```python
from build123d import *

# Parameters (mm, degrees)
F0_R     = 15
F1_DEPTH = 20
F2_W     = 40
F2_H     = 40
F3_DEPTH = 100
F5_D     = 17


with BuildPart() as f1:
    # F0 (on Right) → F1 (new body, symmetric)
    with BuildSketch(Plane.YZ):
        Polygon((-80, -5), (-40, -40), (40, -40), (80, -5), (80, 35), (-80, 35), align=None)
        Circle(F0_R, mode=Mode.SUBTRACT)
    extrude(amount=F1_DEPTH, both=True)

    # F2 (on Right) → F3 (join, symmetric)
    with BuildSketch(Plane.YZ):
        with Locations((-60, 15)):
            Rectangle(F2_W, F2_H)
        with Locations((60, 15)):
            Rectangle(F2_W, F2_H)
    extrude(amount=F3_DEPTH, both=True)

    # F5 (through all)
    with Locations(Plane.XY.offset(35)):
        with Locations((-80, 60), (80, 60), (80, -60), (-80, -60)):
            Hole(F5_D / 2)


solid = f1.part
```
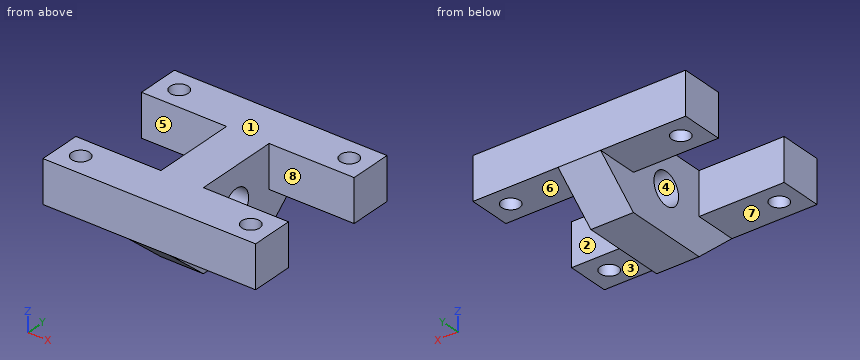
Geometry: final body of the model. Coordinates: model frame, mm. Face numbers are marked on the shaded views. A direction names the side the tool comes from. Round coordinates to 2 decimals unless told otherwise and drop trailing zeros. Order: outer loops, then holes, each group sorted by start corner. A loop starts at its lowest first (then second) coordinate and runs counter-clockwise, first axis right, second up. Notation, with made-up numbers: (34, -5.5) - (44, -5.5) arc R30 cw to (44, 26.5) - close; hole circle Ø1 at (73.25, 82). An arc over 180 degrees is marked (long way). Write item = value, one per line. Start each with the question number.
Q1. Ray query, line 1 (Y direction, x = 80, z = 11); line 2 (Z direction, x = -0.5, y = 0); line 3 (Y direction, x = 70.5, z = 11). Return the intervals inside material, ascending. Write a range as from..to.
Q2. Access query for the marked faces 5, 6, 7 and 8. Directions: +Z, -Z, +X, -X, +Y, -Y. A direction counts if a zero-diameter tool reaches every point of the face in a straight line with its end or side. Return the directions, or none.
Q3. Cut plane D-D on y = 60. Return the cut outline in (x, z), and give its area (3 significant figures).
Q4. Pin query (flat end, axial travel): pin 1 (1.5 mm diameter, centred on y = -38, z = -32, fed in from -X); pin 2 (20 mm diameter, centred on x = -66, y = -65, fed in from -Z); pin 3 (22.5 mm diameter, centred on y = 7, z = 9.5, fed in from +X). Return the tip coordinate at first contact, or that it passes through.
Q5. Pull-direction query (Z, two-part tool) for the marked faces 1, 2, 3 and 4; classes: +Z half, -Z half, draft (parallel to the pull), parting line (faces both ways), or undercut.
Q6. Cut plane A-A on z = 0. Return the cut outline in (x, y).
Q7. Cut plane B-B on y = 0. Return the cut outline in (x, z), and give its area (3 significant figures).
Q8. Cut plane C-C on x = -37. Return the cut outline in (y, z).
Outcome:
q1.line_1 = -80..-68.5, -51.5..-40, 40..51.5, 68.5..80
q1.line_2 = -40..-15, 15..35
q1.line_3 = -80..-40, 40..80
q2.face_5 = +Z, -Z, -X
q2.face_6 = -Z, +X, +Y, -Y
q2.face_7 = -Z, -X, +Y, -Y
q2.face_8 = +Z, -Z, +X
q3.outline = (-100, -5) - (-88.5, -5) - (-88.5, 35) - (-100, 35) - close; (-71.5, -5) - (-20, -5) - (-20, -22.5) - (20, -22.5) - (20, -5) - (71.5, -5) - (71.5, 35) - (-71.5, 35) - close; (88.5, -5) - (100, -5) - (100, 35) - (88.5, 35) - close
q3.area = 7,340 mm^2
q4.pin_1 = -20
q4.pin_2 = -5
q4.pin_3 = 20
q5.face_1 = +Z half
q5.face_2 = draft
q5.face_3 = -Z half
q5.face_4 = undercut
q6.outline = (-100, -80) - (100, -80) - (100, -40) - (20, -40) - (20, -15) - (-20, -15) - (-20, -40) - (-100, -40) - close; (-100, 40) - (-20, 40) - (-20, 15) - (20, 15) - (20, 40) - (100, 40) - (100, 80) - (-100, 80) - close; hole circle Ø17 at (-80, -60); hole circle Ø17 at (-80, 60); hole circle Ø17 at (80, -60); hole circle Ø17 at (80, 60)
q7.outline = (-20, -40) - (20, -40) - (20, -15) - (-20, -15) - close; (-20, 15) - (20, 15) - (20, 35) - (-20, 35) - close
q7.area = 1,800 mm^2
q8.outline = (-80, -5) - (-40, -5) - (-40, 35) - (-80, 35) - close; (40, -5) - (80, -5) - (80, 35) - (40, 35) - close
